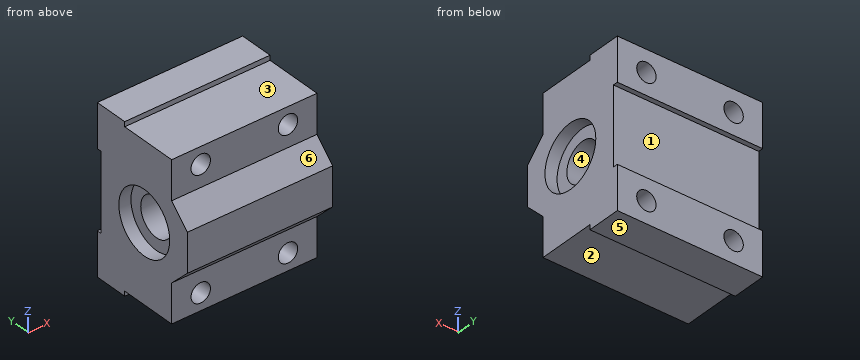
Autodesk Inventor part; units mm, degrees
ref_plane "YZ Plane" through (0, 0, 0) normal (1, 0, 0) x (0, 1, 0)
ref_plane "XZ Plane" through (0, 0, 0) normal (0, 1, 0) x (-1, 0, 0)
ref_plane "XY Plane" through (0, 0, 0) normal (0, 0, 1) x (1, 0, 0)
sketch "Sketch1" plane through (0, 0, 0) normal (1, 0, 0) x (0, 1, 0)
  circle A0 centre (0, 0) radius 4
  line L0 (0, 23.8) -> (0, -23.8)
  line L1 (-15.6, 0) -> (16.6, 0)
  line L2 (11, 17) -> (11, -17)
  line L3 (11, -17) -> (5, -17)
  line L4 (5, -17) -> (5, -16)
  line L5 (5, -16) -> (-7, -16)
  line L6 (-7, -16) -> (-7, -8)
  line L7 (-7, -8) -> (-11, -4)
  line L8 (-11, -4) -> (-11, 4)
  line L9 (-11, 4) -> (-7, 8)
  line L10 (-7, 8) -> (-7, 16)
  line L11 (-7, 16) -> (5, 16)
  line L12 (5, 16) -> (5, 17)
  line L13 (5, 17) -> (11, 17)
  circle A1 centre (0, 0) radius 6.5
  line L14 (11, -12) -> (-7, -12) construction
  line L15 (-7, -14) -> (11, -14) construction
  line L16 (11, -10) -> (-7, -10) construction
  line L17 (11, -17) -> (12, -17)
  line L18 (12, -17) -> (12, -8)
  line L19 (12, -8) -> (11, -8)
  line L20 (11, 17) -> (12, 17)
  line L21 (12, 17) -> (12, 8)
  line L22 (12, 8) -> (11, 8)
  dimension "d0" = 34
  dimension "d1" = 22
  dimension "d2" = 11
  dimension "d3" = 6
  dimension "d4" = 18
  dimension "d5" = 1
  dimension "d6" = 8
  dimension "d7" = 13
  dimension "d9" = 5
  dimension "d10" = 4
  dimension "d11" = 4
  dimension "d12" = 8
  dimension "d17" = 1
extrude "Extrusion1" add sketch "Sketch1" along normal mid plane 30 contours A1 L0 L11 L12 L13 L2 L1 | L1 L2 L3 L4 L5 L0 A1 | A1 L1 L8 L9 L10 L11 L0 | L0 L5 L6 L7 L8 L1 A1 | L2 L20 L21 L22 | L19 L18 L17 L2
extrude "Extrusion2" add sketch "Sketch1" along normal mid plane 25 contours L1 A1 L0 A0 | A0 L0 A1 L1 | A0 L1 A1 L0 | L0 A1 L1 A0
sketch "Sketch2" plane through (-15, 12, 17) normal (0, 1, 0) x (1, 0, 0)
  line L0 (30, 0) -> (0, 0)
  line L1 (30, 9) -> (30, 0)
  line L2 (0, 9) -> (30, 9)
  line L3 (0, 0) -> (0, 9)
  line L4 (0, 25) -> (30, 25)
  line L5 (30, 34) -> (30, 25)
  line L6 (0, 34) -> (30, 34)
  line L7 (0, 25) -> (0, 34)
  line L8 (36, 17) -> (-6, 17)
  line L9 (15, 40.8) -> (15, -6.8)
  circle A0 centre (6, 4.5) radius 2
  circle A1 centre (24, 4.5) radius 2
  circle A2 centre (6, 29.5) radius 2
  circle A3 centre (24, 29.5) radius 2
  point P0 (15, 17)
  dimension "d18" = 4.5
  dimension "d19" = 18
  dimension "d20" = 4
extrude "Extrusion3" cut sketch "Sketch2" against normal up to next contours A0 | A1 | A2 | A3
properties part number "Linear Bearing Platform Small" material "Aluminum 6061"
Work out the finished part from the listing and answer in its coordinate system (mm). Face numbers are marked on the shaded views. A direction names the side the tool comes from. Round coordinates to 2 decimals unless told otherwise and drop trailing zeros. Loops run counter-clockwise (first coordinate to the right, second up) from the corner with the lowest first, then second, coordinate; pieces in that order, holes last. Notation, with made-up numbers: (-9, 49.5) - (-1, 49.5) arc R16 cw to (-1, 64.5) - close; hole circle Ø9 at (13.5, 38). An arc over 180 degrees is marked (long way). One line per item, written item: value.
Q1. For the marked faces 1, 2 and 3, determine the directions among +Z, -Z, +X, -X, +Y, -Y from which every point of the face is accessible in a straight line to the end or side of a thin tool.
Check values:
face 1: +X, -X, +Y
face 2: -Z, +X, -X, -Y
face 3: +Z, +X, -X, -Y
Q2. The mould has two halves that part along Z. Classify the marked faces 4, 5 and 6: +Z half, -Z half, draft (parallel to the pull), parting line (faces both ways), or undercut.
Check values:
face 4: undercut
face 5: -Z half
face 6: +Z half
Q3. Each of these flat-tipped pins is pushed along its axis until it touches: pin 1 Ø6 at (x, y) = (6, -3) entering from -Z; pin 2 Ø12 at (x, z) = (-2, 0.5) entering from +Y; pin 3 Ø2.5 at (x, z) = (-6.5, -12.5) entering from -Y. Where does it stop, or does it pass through?
Check values:
pin 1: z = -16
pin 2: y = 11
pin 3: y = -7
Q4. Find section D-D on z = -6. Give the vertices of the cut face in (x, y).
Check values:
outline: (-15, -9) - (15, -9) - (15, -2.5) - (12.5, -2.5) - (12.5, 2.5) - (15, 2.5) - (15, 11) - (-15, 11) - (-15, 2.5) - (-12.5, 2.5) - (-12.5, -2.5) - (-15, -2.5) - close
Q5. Find section B-B on z = -12.5. Give the vertices of the cut face in (x, y), and give its area (3 significant figures).
Check values:
outline: (-15, -7) - (-11, -7) - (-11, 12) - (-15, 12) - close; (-7, -7) - (7, -7) - (7, 12) - (-7, 12) - close; (11, -7) - (15, -7) - (15, 12) - (11, 12) - close
area: 418 mm2
Q6. Find section C-C on y = 6. Give the vertices of the cut face in (x, z), and give its area (3 significant figures).
Check values:
outline: (-15, -17) - (15, -17) - (15, -2.5) - (12.5, -2.5) - (12.5, 2.5) - (15, 2.5) - (15, 17) - (-15, 17) - (-15, 2.5) - (-12.5, 2.5) - (-12.5, -2.5) - (-15, -2.5) - close; hole circle Ø4 at (-9, -12.5); hole circle Ø4 at (-9, 12.5); hole circle Ø4 at (9, -12.5); hole circle Ø4 at (9, 12.5)
area: 945 mm2
Q7. Find section A-A on x = -9. Give the vertices of the cut face in (y, z), and give its area (3 significant figures).
Check values:
outline: (-11, -4) - (-7, -8) - (-7, -10.5) - (12, -10.5) - (12, -8) - (11, -8) - (11, 8) - (12, 8) - (12, 10.5) - (-7, 10.5) - (-7, 8) - (-11, 4) - close; (-7, -16) - (5, -16) - (5, -17) - (12, -17) - (12, -14.5) - (-7, -14.5) - close; (-7, 14.5) - (12, 14.5) - (12, 17) - (5, 17) - (5, 16) - (-7, 16) - close; hole circle Ø8 at (0, 0)
area: 452 mm2
Q8. Straight lines are drawn through the part: probe 1 along Y at (x, z) = (13.25, 0); probe 2 along X at (y, z) = (-2, -12.5); probe 3 along Z at (x, y) = (-9, 5.25). For each, find the intervals that lie inside material, in ascending order.
Check values:
probe 1: -11 to -6.5, 6.5 to 11
probe 2: -15 to -11, -7 to 7, 11 to 15
probe 3: -17 to -14.5, -10.5 to 10.5, 14.5 to 17
